```python
from build123d import *

# Parameters (mm, degrees)
F1_DEPTH  = 25.4
F2_R      = 6.35
F3_DEPTH  = 51.60825547
F5_DEPTH  = 51.60825547
F6_R      = 9.122141835
F7_DEPTH  = 12.701
F8_R      = 6.35
F9_DEPTH  = 12.701
F11_DEPTH = 12.701
F13_DEPTH = 12.701


with BuildPart() as f1:
    # F0 (on Front) → F1 (new body)
    with BuildSketch(Plane.XZ):
        Polygon((-70.854865197, 12.7), (-96.254865197, 12.7), (-96.254865197, 0), (-13.704865197, 0), (-13.704865197, 12.7), (-44.647609727, 12.7), (-44.647609727, 44.45), (-70.047609727, 44.45), align=None)
    extrude(amount=F1_DEPTH)

    # F2 (on face) → F3 (cut, through all)
    with BuildSketch(Plane.YZ.offset(-44.647609727)):
        with Locations((-12.7, 31.75)):
            Circle(F2_R)
    extrude(amount=-F3_DEPTH, mode=Mode.SUBTRACT)

    # F4 (on face) → F5 (cut, through all)
    with BuildSketch(Plane.YZ.offset(-44.647609727)):
        with BuildLine():
            ThreePointArc((-25.4, 35.7528030872), (-20.7098485948, 41.9702258596), (-13.3271264447, 44.45))
            Line((-13.3271264447, 44.45), (-25.4, 44.45))
            Line((-25.4, 44.45), (-25.4, 35.7528030872))
        make_face()
        with BuildLine():
            Line((0, 44.45), (-11.4556124951, 44.45))
            ThreePointArc((-11.4556124951, 44.45), (-4.4379972961, 41.9413380989), (0, 35.9543114901))
            Line((0, 35.9543114901), (0, 44.45))
        make_face()
    extrude(amount=-F5_DEPTH, mode=Mode.SUBTRACT)

    # F6 (on face) → F7 (cut, through all)
    with BuildSketch(Plane.XY.offset(12.7)):
        with Locations((-29.176237462, -12.5456847349)):
            Circle(F6_R)
    extrude(amount=-F7_DEPTH, mode=Mode.SUBTRACT)

    # F8 (on face) → F9 (cut, through all)
    with BuildSketch(Plane.XY.offset(12.7)):
        with Locations((-83.554865197, -12.7)):
            Circle(F8_R)
    extrude(amount=-F9_DEPTH, mode=Mode.SUBTRACT)

    # F10 (on face) → F11 (cut, through all)
    with BuildSketch(Plane.XY.offset(12.7)):
        with BuildLine():
            ThreePointArc((-96.254865197, -12.7), (-92.5351213181, -3.7197438789), (-83.554865197, 0))
            Line((-83.554865197, 0), (-96.254865197, 0))
            Line((-96.254865197, 0), (-96.254865197, -12.7))
        make_face()
        with BuildLine():
            ThreePointArc((-83.554865197, -25.4), (-92.5351213181, -21.6802561211), (-96.254865197, -12.7))
            Line((-96.254865197, -12.7), (-96.254865197, -25.4))
            Line((-96.254865197, -25.4), (-83.554865197, -25.4))
        make_face()
    extrude(amount=-F11_DEPTH, mode=Mode.SUBTRACT)

    # F12 (on face) → F13 (cut, through all)
    with BuildSketch(Plane.XY.offset(12.7)):
        with BuildLine():
            ThreePointArc((-24.1288895467, 0), (-16.6844564555, -4.4358743894), (-13.704865197, -12.5733556693))
            Line((-13.704865197, -12.5733556693), (-13.704865197, 0))
            Line((-13.704865197, 0), (-24.1288895467, 0))
        make_face()
        with BuildLine():
            ThreePointArc((-13.704865197, -12.8266443307), (-16.6844564555, -20.9641256106), (-24.1288895467, -25.4))
            Line((-24.1288895467, -25.4), (-13.704865197, -25.4))
            Line((-13.704865197, -25.4), (-13.704865197, -12.8266443307))
        make_face()
    extrude(amount=-F13_DEPTH, mode=Mode.SUBTRACT)


solid = f1.part
```
Read the model definition and answer for the solid it produces. Units are mm, in the model's axes. A direction names the side the tool comes from. Round coordinates to 2 decimals unless told otherwise and drop trailing zeros. Loops run counter-clockwise (first coordinate to the right, second up) from the corner with the lowest first, then second, coordinate; pieces in that order, holes last. Notation, with made-up numbers: (-10.5, 5) -> (48.5, 5) arc R19 ccw to (48.5, 38) -> close; hole circle Ø9 at (43.25, 1). An arc over 180 degrees is marked (long way). One line per item, written item: value.
1) For faces 4 (the face through (-44.648, -13, 25)), 5 (the face through (-57.425, -6.643, 33.657)), 6 (the face through (-77.7, -9.7, 12.7)), determine the directions among +Z, -Z, +X, -X, +Y, -Y from which every point of the face is accessible in a straight line to the end or side of a thin tool.
Answer list:
face 4: +Z, +X, +Y, -Y
face 5: +X, -X
face 6: +Z, -X, +Y, -Y
2) Flat-ended cylindrical pins translate along their axes: P1, Ø12, axis at y = -9.5, z = 9, coming from the -X side; P2, Ø1.5, axis at y = -3, z = 29.5, coming from the +X side; P3, Ø7.5, axis at x = -78.5, y = -11, coming from the +Z side; P4, Ø6, axis at y = -15, z = 31, coming from the -X side. Find the tip coordinate at first contact, or state that the pin passes through.
Answer list:
P1: stops at x = -96.25
P2: stops at x = -44.65
P3: stops at z = 12.7
P4: passes through
3) A cutting plane is placed at B-B (x = -52.5). Determine the outline of the cut face in (y, z).
Answer list:
outline: (-25.4, 0) -> (0, 0) -> (0, 35.95) arc R12.83 ccw to (-11.46, 44.45) -> (-13.33, 44.45) arc R13.17 ccw to (-25.4, 35.75) -> close; hole circle Ø12.7 at (-12.7, 31.75)
4) Consider L1, parallel to X at y = -12.5, z = 6.5; L2, parallel to Z at x = -58.5, y = -13; L3, parallel to Y at x = -52.25, z = 31.75. Determine where each line is inside the solid, lowest interval first. Write a range as [from, to].
Answer list:
L1: x = [-96.25, -89.9], [-77.21, -38.3], [-20.05, -13.71]
L2: z = [0, 25.41], [38.09, 44.45]
L3: y = [-25.4, -19.05], [-6.35, 0]
5) A cutting plane is placed at A-A (y = -16.75). Determine the outline of the cut face in (x, z), and give its area (3 significant figures).
Answer list:
outline: (-95.59, 0) -> (-88.45, 0) -> (-88.45, 12.7) -> (-95.59, 12.7) -> close; (-78.66, 0) -> (-37.27, 0) -> (-37.27, 12.7) -> (-44.65, 12.7) -> (-44.65, 26.86) -> (-70.49, 26.86) -> (-70.85, 12.7) -> (-78.66, 12.7) -> close; (-70.25, 36.64) -> (-44.65, 36.64) -> (-44.65, 43.91) -> (-70.06, 43.91) -> close; (-21.08, 0) -> (-14.35, 0) -> (-14.35, 12.7) -> (-21.08, 12.7) -> close
area: 1,260 mm²
6) The mould has two halves that part along Y. Classify faces 1 (the face through (-89.9, -12.42, 6.44)), 2 (the face through (-39, -13, 12.7)), 3 (the face through (-54, 0, 14)): pulls with the +Y half, pulls with the -Y half, needs draft (parallel to the pull), parting line crosses it, or undercut.
Answer list:
face 1: undercut
face 2: needs draft
face 3: pulls with the +Y half
7) A cutting plane is placed at D-D (z = 31.75). Determine the outline of the cut face in (x, y).
Answer list:
outline: (-70.37, -25.4) -> (-44.65, -25.4) -> (-44.65, -19.05) -> (-70.37, -19.05) -> close; (-70.37, -6.35) -> (-44.65, -6.35) -> (-44.65, 0) -> (-70.37, 0) -> close
8) A cutting plane is placed at C-C (z = 6). Determine the outline of the cut face in (x, y), and give its area (3 significant figures).
Answer list:
outline: (-83.55, -25.4) -> (-24.13, -25.4) arc R12.95 ccw to (-13.7, -12.83) -> (-13.7, -12.57) arc R12.95 ccw to (-24.13, 0) -> (-83.55, 0) arc R12.7 ccw to start; hole circle Ø12.7 at (-83.55, -12.7); hole circle Ø18.24 at (-29.18, -12.55)
area: 1,570 mm²
